Build history of the part. All positions in model axes, mm. A direction names the side the tool comes from. Give positions to 0.01 mm unless a question says otherwise; leave off trailing zeros. Loops run counter-clockwise (first coordinate to the right, second up) from the corner with the lowest first, then second, coordinate; pieces in that order, holes last. Notation, with made-up numbers: M 14,42 L 68,42 A24 cw 68,62 Z; hole C 7.25,63.25 d3. An arc over 180 degrees is marked long. Answer as a JSON object with one key per item and string values. Group by question number.
1. Slice it at B-B (x = 0). List the corners of the cut face in (y, z).
2. Drop flat-ended pins along their axis: pin 1 Ø10 at (x, z) = (28, 26) entering from +Y; pin 2 Ø2 at (y, z) = (4, -42.5) entering from +X. Give the stop position or say it passes through.
3. Slice it at D-D (z = -38.5). Give the number of separate pieces and of enclosed holes in the cut face, then the cut area to 3 significant figures.
4. Slice it at A-A (z = 53.5). List the corners of the cut face in (x, y) (3 decimals), then the cut area to 3 significant figures.
5. 3-axis set-ups, long thin cutter, end or side, ignore diameter. For faces 1 (the face through (-1, 5, -17)), 2 (the face through (0, -1, 45)): which of +Z, -Z, +X, -X, +Y, -Y reach the whole face in a straight line?
6. Mould opens along X. For faces 3 (the face through (40.12, -1.479, -39.753)), 4 (the face through (1, -3, -1)), 5 (the face through (-47.15, -1.48, -61.99)) say: released by +X, released by -X, zero draft, split by the parting line, or undercut.
7. Slice it at C-C (z = 38.5). List the corners of the cut face in (x, y) (3 decimals).
8. Drill centre lines: line 1 along X through (y, z) = (-1.6, 38.5) (3 decimals); line 2 along X through (y, z) = (-0.25, -37.5); line 3 along Z through (x, y) = (3.5, -1.5). Where is each one in solid material? Low to high. Write a range as [from, to].
from build123d import *

# Parameters (mm, degrees)
SKETCH1_R           = 1.6
SKETCH1_R_2         = 1.7
BOSS_EXTRUDE1_DEPTH = 3
SKETCH2_R           = 40.5
BOSS_EXTRUDE2_DEPTH = 5
BOSS_EXTRUDE2_TAPER = 5
FILLET1_R           = 2


with BuildPart() as part:
    # Sketch1 → Boss-Extrude1 (new body)
    with BuildSketch(Plane(origin=(0, 0, 0), x_dir=(1, 0, 0), z_dir=(0, 1, 0))):
        with BuildLine():
            Line((40, -65), (-40, -65))
            ThreePointArc((-40, -65), (-47.071067812, -62.071067812), (-50, -55))
            Line((-50, -55), (-50, 55))
            ThreePointArc((-50, 55), (-47.071067812, 62.071067812), (-40, 65))
            Line((-40, 65), (40, 65))
            ThreePointArc((40, 65), (47.071067812, 62.071067812), (50, 55))
            Line((50, 55), (50, -55))
            ThreePointArc((50, -55), (47.071067812, -62.071067812), (40, -65))
        make_face()
        with Locations(Location((21.475, -38.5, 0), (0, 0, 270))):
            Circle(SKETCH1_R, mode=Mode.SUBTRACT)
        with Locations(Location((21.475, -53.5, 0), (0, 0, 270))):
            Circle(SKETCH1_R, mode=Mode.SUBTRACT)
        with Locations(Location((-21.475, -38.5, 0), (0, 0, 270))):
            Circle(SKETCH1_R, mode=Mode.SUBTRACT)
        with Locations(Location((-21.475, -53.5, 0), (0, 0, 270))):
            Circle(SKETCH1_R, mode=Mode.SUBTRACT)
        with Locations(Location((0, -29, 0), (0, 0, 270))):
            Circle(SKETCH1_R_2, mode=Mode.SUBTRACT)
        with Locations(Location((-38.97114317, 38.5, 0), (0, 0, 270))):
            Circle(SKETCH1_R_2, mode=Mode.SUBTRACT)
        with Locations(Location((38.97114317, 38.5, 0), (0, 0, 270))):
            Circle(SKETCH1_R_2, mode=Mode.SUBTRACT)
        with BuildLine():
            Line((3, -57), (-3, -57))
            ThreePointArc((-3, -57), (-4.414213562, -56.414213562), (-5, -55))
            Line((-5, -55), (-5, -47))
            ThreePointArc((-5, -47), (-4.414213562, -45.585786438), (-3, -45))
            Line((-3, -45), (3, -45))
            ThreePointArc((3, -45), (4.414213562, -45.585786438), (5, -47))
            Line((5, -47), (5, -55))
            ThreePointArc((5, -55), (4.414213562, -56.414213562), (3, -57))
        make_face(mode=Mode.SUBTRACT)
    extrude(amount=-BOSS_EXTRUDE1_DEPTH)

    # Sketch2 → Boss-Extrude2 (add)
    with BuildSketch(Plane(origin=(0, 0, 0), x_dir=(1, 0, 0), z_dir=(0, 1, 0))):
        with Locations((0, 16)):
            Circle(SKETCH2_R)
    extrude(amount=BOSS_EXTRUDE2_DEPTH, taper=BOSS_EXTRUDE2_TAPER)

    # Fillet1
    fillet1_edges = [part.edges().sort_by_distance(p)[0] for p in [
        (-40.062556682, 5, -16),
    ]]
    fillet(fillet1_edges, radius=FILLET1_R)


solid = part.part
Established:
{
 "1": {"outline": "M -3,-65 L 0,-65 L 0,-56.5 L 3.17,-56.22 A2 ccw 5,-54.23 L 5,22.23 A2 ccw 3.17,24.22 L 0,24.5 L 0,27.3 L -3,27.3 Z; M -3,30.7 L 0,30.7 L 0,45 L -3,45 Z; M -3,57 L 0,57 L 0,65 L -3,65 Z"},
 "2": {"pin 1": "stops at y = 0", "pin 2": "stops at x = 30.93"},
 "3": {"separate pieces": "3", "enclosed holes": "0", "area": "612 mm^2"},
 "4": {"outline": "M -50,-3 L -23.075,-3 L -23.075,0 L -50,0 Z; M -19.875,-3 L -5,-3 L -5,0 L -19.875,0 Z; M 5,-3 L 19.875,-3 L 19.875,0 L 5,0 Z; M 23.075,-3 L 50,-3 L 50,0 L 23.075,0 Z", "area": "251 mm^2"},
 "5": {"face 1": "+Z, -Z, +X, -X, +Y", "face 2": "+Y, -Y"},
 "6": {"face 3": "undercut", "face 4": "zero draft", "face 5": "released by -X"},
 "7": {"outline": "M -50,-3 L -23.075,-3 L -23.075,0 L -50,0 Z; M -19.875,-3 L 19.875,-3 L 19.875,0 L -19.875,0 Z; M 23.075,-3 L 50,-3 L 50,0 L 23.075,0 Z"},
 "8": {"line 1": "x = [-50, -23.075], [-19.875, 19.875], [23.075, 50]", "line 2": "x = [-50, -40.35], [-37.6, 37.6], [40.35, 50]", "line 3": "z = [-65, 45.06], [56.94, 65]"}
}
